```python
from build123d import *

# Parameters (mm, degrees)
SKETCH2_W           = 95.25
SKETCH2_H           = 66.802
SKETCH2_W_2         = 82.296
SKETCH2_H_2         = 54.102
BOSS_EXTRUDE1_DEPTH = 10.16
SKETCH3_R           = 1.9939
SKETCH3_R_2         = 1.8669
CUT_EXTRUDE1_DEPTH  = 7.62
SKETCH4_W           = 6.35
SKETCH4_H           = 6.2484
CUT_EXTRUDE2_DEPTH  = 2.54
SKETCH6_W           = 7.62
SKETCH6_H           = 6.2484
SKETCH6_W_2         = 6.35
CUT_EXTRUDE3_DEPTH  = 2.54
FILLET1_R           = 2.54


with BuildPart() as part:
    # Sketch2 → Boss-Extrude1 (new body)
    with BuildSketch(Plane(origin=(0, 0, 0), x_dir=(1, 0, 0), z_dir=(0, 1, 0))):
        Rectangle(SKETCH2_W, SKETCH2_H)
        Rectangle(SKETCH2_W_2, SKETCH2_H_2, mode=Mode.SUBTRACT)
    extrude(amount=BOSS_EXTRUDE1_DEPTH)

    # Sketch3 → Cut-Extrude1 (cut)
    with BuildSketch(Plane.XZ):
        with Locations((-44.45, 30.48)):
            Circle(SKETCH3_R)
        with Locations((44.45, 30.48)):
            Circle(SKETCH3_R)
        with Locations((44.45, -30.48)):
            Circle(SKETCH3_R_2)
        with Locations((-44.45, -30.48)):
            Circle(SKETCH3_R)
    extrude(amount=-CUT_EXTRUDE1_DEPTH, mode=Mode.SUBTRACT)

    # Sketch4 → Cut-Extrude2 (cut)
    with BuildSketch(Plane(origin=(0, 0, 27.051), x_dir=(-1, 0, 0), z_dir=(0, 0, -1))):
        with Locations((27.178, 3.1242)):
            Rectangle(SKETCH4_W, SKETCH4_H)
        with Locations((-27.178, 3.1242)):
            Rectangle(SKETCH4_W, SKETCH4_H)
    extrude(amount=-CUT_EXTRUDE2_DEPTH, mode=Mode.SUBTRACT)

    # Sketch6 → Cut-Extrude3 (cut)
    with BuildSketch(Plane.ZY.offset(-41.148)):
        with Locations((-23.241, 3.1242)):
            Rectangle(SKETCH6_W, SKETCH6_H)
        with Locations((23.241, 3.1242)):
            Rectangle(SKETCH6_W, SKETCH6_H)
        with Locations((0, 3.1242)):
            Rectangle(SKETCH6_W_2, SKETCH6_H)
    extrude(amount=-CUT_EXTRUDE3_DEPTH, mode=Mode.SUBTRACT)

    # Fillet1
    fillet1_edges = [part.edges().sort_by_distance(p)[0] for p in [
        (47.625, 10.16, 0),
        (0, 10.16, -33.401),
        (-47.625, 10.16, 0),
        (-47.625, 5.08, -33.401),
        (47.625, 5.08, -33.401),
        (47.625, 5.08, 33.401),
        (-47.625, 5.08, 33.401),
        (0, 10.16, 33.401),
    ]]
    fillet(fillet1_edges, radius=FILLET1_R)


solid = part.part
```
Input: part model. Units: mm. Frame: model coordinates. A direction names the side the tool comes from. Coordinates: 2 decimals unless noted, no trailing zeros. Write each loop counter-clockwise with the first axis right and the second up, starting at its lowest first coordinate (ties: lowest second). Pieces come first, ordered by that corner, then holes. Notation, with made-up numbers: (11.25, 82.5) - (30.25, 82.5) arc R24 cw to (30.25, 107.5) - close; hole circle Ø4 at (53, -32). An arc over 180 degrees is marked (long way). Put each result on its own line as item: value. Start each with the question number.
1) Mould query, pull axis Z, two halves, no side actions, for faces 1 (the face through (-1, 4, -33.401)), 2 (the face through (27, 6.248, 28)), 3 (the face through (0.631, 9.436, 32.637)), 4 (the face through (-46.901, 9.396, -0.432)). Classes: pulls with the +Z half, pulls with the -Z half, needs draft (parallel to the pull), parting line crosses it, or undercut.
2) Reachability of faces 5 (the face through (-41.148, 5, 0)), 6 (the face through (42, 3, -3.175)), 7 (the face through (-46.9, 3.86, -32.64)) from +Z, -Z, +X, -X, +Y, -Y: full face, straight path, thin tool, end or side. Return the list, or none.
3) Cut plane D-D (z = 7). Return the cut outline in (x, y) (3 decimals).
4) Ray query, L1, parallel to Z at x = 44.45, y = 1.75; L2, parallel to Z at x = -44.45, y = 4.5; L3, parallel to Z at x = -2, y = 6.75. Return the intervals inside material, ascending.
5) Cut plane B-B (y = 1.75). State how many separate pieces and enclosed holes the cut face has, plus the area to 3 significant figures.
6) Cut plane C-C (x = -19). Return the cut outline in (y, z).
7) Contact query for flat-ended pins moving along their axis: pin 1 (4 mm diameter, centred on x = 44, z = -30, fed in from -Y); pin 2 (3.5 mm diameter, centred on x = 44.45, z = -30.48, fed in from -Y); pin 3 (3 mm diameter, centred on x = 42, z = -25, fed in from -Y). Output: stop coordinate, or through.
8) Cut plane A-A (z = -25.5). Return the cut outline in (x, y) (3 decimals).
Resolved:
1. face 1: pulls with the -Z half
1. face 2: undercut
1. face 3: pulls with the +Z half
1. face 4: needs draft
2. face 5: +Y, -Y
2. face 6: -Y
2. face 7: -Z, -X, +Y, -Y
3. outline: (-47.625, 0) - (-41.148, 0) - (-41.148, 10.16) - (-45.085, 10.16) arc R2.54 ccw to (-47.625, 7.62) - close; (41.148, 0) - (47.625, 0) - (47.625, 7.62) arc R2.54 ccw to (45.085, 10.16) - (41.148, 10.16) - close
4. L1: z = -33.4 to -32.35, -28.61 to 28.49, 32.47 to 33.4
4. L2: z = -33.4 to -32.47, -28.49 to 28.49, 32.47 to 33.4
4. L3: z = -33.4 to -27.05, 27.05 to 33.4
5. separate pieces: 1
5. enclosed holes: 5
5. area: 1,770 mm2
6. outline: (0, -33.4) - (7.62, -33.4) arc R2.54 ccw to (10.16, -30.86) - (10.16, -27.05) - (0, -27.05) - close; (0, 27.05) - (10.16, 27.05) - (10.16, 30.86) arc R2.54 ccw to (7.62, 33.4) - (0, 33.4) - close
7. pin 1: stops at y = 0
7. pin 2: stops at y = 7.62
7. pin 3: stops at y = 6.25
8. outline: (-47.625, 0) - (-41.148, 0) - (-41.148, 10.16) - (-45.085, 10.16) arc R2.54 ccw to (-47.625, 7.62) - close; (41.148, 6.248) - (43.688, 6.248) - (43.688, 0) - (47.625, 0) - (47.625, 7.62) arc R2.54 ccw to (45.085, 10.16) - (41.148, 10.16) - close
